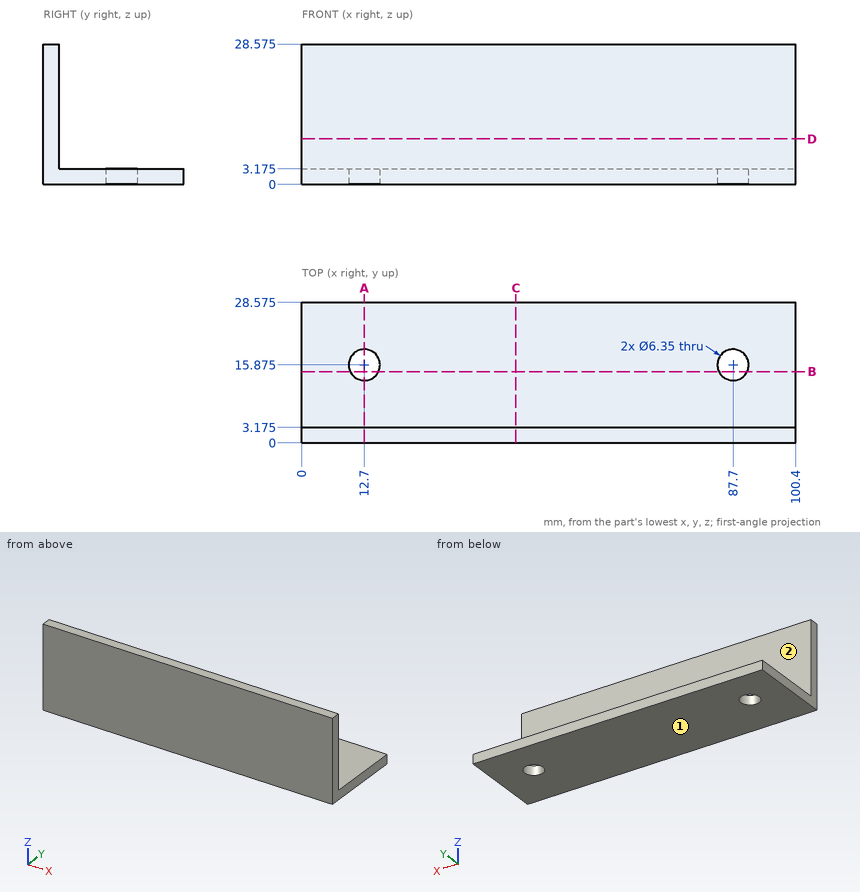
Design review of the part shown in the three views and the two pictorial views. Dimensions are in mm from the part's minimum x, y and z. A direction names the side the tool comes from. Round coordinates to 2 decimals unless told otherwise and drop trailing zeros. Order: outer loops, then holes, each group sorted by start corner. A loop starts at its lowest first (then second) coordinate and runs counter-clockwise, first axis right, second up.
Q1. We need section C-C, the plane x = 43.5. Give the boundary of the cut face in (y, z) (3 decimals), plus the area to 3 significant figures.
Findings below:
outline: (0, 0) - (28.575, 0) - (28.575, 3.175) - (3.175, 3.175) - (3.175, 28.575) - (0, 28.575) - close
area: 171 mm2
Q2. Insertion check: P1, Ø3, axis at x = 38.5, y = 5, coming from the -Z side; P2, Ø5, axis at x = 14.5, y = 16, coming from the +Z side (3 decimals); P3, Ø12, axis at y = 11.5, z = 22, coming from the +X side; P4, Ø1.5, axis at x = 69, z = 19.5, coming from the +Y side (3 decimals). Each pin has a flat end and moves straight along its axis. Give the tip position at first contact, or say it passes through.
Findings below:
P1: stops at z = 0
P2: stops at z = 3.175
P3: passes through
P4: stops at y = 3.175
Q3. Wall thickness on line 1 (Y direction, x = 12.7, z = 0.7) (3 decimals); line 2 (Z direction, x = 9, y = 6.75) (3 decimals): over which ranges is each line inside the solid? List them lowest first.
Findings below:
line 1: y = 0 to 12.7, 19.05 to 28.575
line 2: z = 0 to 3.175
Q4. We need section B-B, the plane y = 14.5. Give the boundary of the cut face in (x, z) (3 decimals).
Findings below:
outline: (0, 0) - (9.838, 0) - (9.838, 3.175) - (0, 3.175) - close; (15.562, 0) - (84.838, 0) - (84.838, 3.175) - (15.562, 3.175) - close; (90.562, 0) - (100.4, 0) - (100.4, 3.175) - (90.562, 3.175) - close
Q5. We need section A-A, the plane x = 12.7. Give the boundary of the cut face in (y, z) (3 decimals), plus the area to 3 significant figures.
Findings below:
outline: (0, 0) - (12.7, 0) - (12.7, 3.175) - (3.175, 3.175) - (3.175, 28.575) - (0, 28.575) - close; (19.05, 0) - (28.575, 0) - (28.575, 3.175) - (19.05, 3.175) - close
area: 151 mm2
Q6. Machinability: for the marked faces 1 and 2, which of the approach directions +Z, -Z, +X, -X, +Y, -Y give a long, thin tool a straight path to every point of the face, cutting with its end or side? Answer none if there is none.
Findings below:
face 1: -Z, +X, -X, +Y, -Y
face 2: +Z, +X, -X, +Y
Q7. We need section D-D, the plane z = 9.25. Give the boundary of the cut face in (x, y) (3 decimals), plus the area to 3 significant figures.
Findings below:
outline: (0, 0) - (100.4, 0) - (100.4, 3.175) - (0, 3.175) - close
area: 319 mm2
